from build123d import *

# Parameters (mm, degrees)
F1_DEPTH = 5
F2_DEPTH = 15
F3_D     = 1.25


with BuildPart() as f1:
    # F0 (on Front) → F1 (new body)
    with BuildSketch(Plane.XZ):
        with BuildLine():
            ThreePointArc((6.4951905284, -3.75), (7.2444436972, -1.9411428383), (7.5, 0))
            ThreePointArc((7.5, 0), (5.3033008589, 5.3033008589), (0, 7.5))
            Line((0, 7.5), (0, 0))
            Line((0, 0), (6.4951905284, -3.75))
        make_face()
        with BuildLine():
            Line((0, 0), (0, 7.5))
            ThreePointArc((0, 7.5), (-6.4951905284, 3.75), (-6.4951905284, -3.75))
            Line((-6.4951905284, -3.75), (0, 0))
        make_face()
        with BuildLine():
            ThreePointArc((6, -4.5), (6.2588394759, -4.1324240362), (6.4951905284, -3.75))
            Line((6.4951905284, -3.75), (0, 0))
            Line((0, 0), (-6.4951905284, -3.75))
            ThreePointArc((-6.4951905284, -3.75), (-6.2588394759, -4.1324240362), (-6, -4.5))
            Line((-6, -4.5), (6, -4.5))
        make_face()
    extrude(amount=F1_DEPTH)

    # F0 (on Front) → F2 (join)
    with BuildSketch(Plane.XZ):
        with BuildLine():
            ThreePointArc((0, -7.5), (3.3541019662, -6.7082039325), (6, -4.5))
            Line((6, -4.5), (-6, -4.5))
            ThreePointArc((-6, -4.5), (-3.3541019662, -6.7082039325), (0, -7.5))
        make_face()
        with BuildLine():
            Line((6, -7.5), (6, -4.5))
            ThreePointArc((6, -4.5), (3.3541019662, -6.7082039325), (0, -7.5))
            Line((0, -7.5), (6, -7.5))
        make_face()
        with BuildLine():
            ThreePointArc((0, -7.5), (-3.3541019662, -6.7082039325), (-6, -4.5))
            Line((-6, -4.5), (-6, -7.5))
            Line((-6, -7.5), (0, -7.5))
        make_face()
    extrude(amount=F2_DEPTH)

    # F3 (through all)
    with Locations(Plane(origin=(0, 0, 0), x_dir=(1, 0, 0), z_dir=(0, 1, 0))):
        with Locations((3.4641016151, 2), (-3.4641016151, 2), (0, -4.5)):
            Hole(F3_D / 2)


solid = f1.part
Input: part model. Units: mm. Frame: model coordinates. A direction names the side the tool comes from. Give positions to 0.01 mm unless a question says otherwise; leave off trailing zeros. Write each loop counter-clockwise with the first axis right and the second up, starting at its lowest first coordinate (ties: lowest second). Pieces come first, ordered by that corner, then holes. Notation, with made-up numbers: M 72,-27.75 L 111,-27.75 A6 ccw 111,-20.75 Z; hole C -29,-4 d10. An arc over 180 degrees is marked long. Write item = value, one per line. Start each with the question number.
1) Material intervals for line 1 along X through (y, z) = (-1.25, -1.5); line 2 along X through (y, z) = (-5.5, -6.25); line 3 along Y through (x, z) = (-2.25, 6.5), sorted ascending. Write a range as [from, to].
2) Draft query along Z for faces 1 (the flat face through (0, -10, -4.5)), 2 (the cylindrical face through (-0.596, -2.535, 4.312)), 3 (the flat face through (0, -5, 2)). Return one class per face: +Z half, -Z half, draft (parallel to the pull), parting line (faces both ways), or undercut.
3) Cut plane C-C on z = -2. Return the cut outline in (x, y).
4) Cut plane D-D on y = -7.25. Return the cut outline in (x, z).
5) First-contact query: pin 1 Ø4 at (y, z) = (-3.5, -5) entering from -X; pin 2 Ø2 at (x, z) = (-2.5, 1.5) entering from -Y; pin 3 Ø4 at (y, z) = (-8.5, 4) entering from -X; pin 4 Ø0.9 at (y, z) = (-6.5, -6) entering from +X. Flat tips, straight axial feed; report the tip coordinate or a pass-through.
6) Cut plane A-A on z = 4.5. Return the cut outline in (x, y) (3 decimals).
7) Reachability of faces 4 (the flat face through (6, -7, -6)), 5 (the flat face through (0, 0, 0)), 6 (the flat face through (-6, -7, -6)) from +Z, -Z, +X, -X, +Y, -Y: full face, straight path, thin tool, end or side. Return the list, or none.
8) Cut plane B-B on y = -1.25. Return the cut outline in (x, z) (3 decimals), then the cut area to 3 significant figures.
Solved:
q1.line_1 = [-7.35, -3.84], [-3.09, 3.09], [3.84, 7.35]
q1.line_2 = [-6, 6]
q1.line_3 = [-5, 0]
q2.face_1 = +Z half
q2.face_2 = undercut
q2.face_3 = draft
q3.outline = M -7.23,-5 L -4.09,-5 L -4.09,0 L -7.23,0 Z; M -2.84,-5 L 2.84,-5 L 2.84,0 L -2.84,0 Z; M 4.09,-5 L 7.23,-5 L 7.23,0 L 4.09,0 Z
q4.outline = M -6,-7.5 L 6,-7.5 L 6,-4.5 L -6,-4.5 Z
q5.pin_1 = -6.87
q5.pin_2 = -5
q5.pin_3 = through
q5.pin_4 = 6
q6.outline = M -6,-5 L -0.625,-5 L -0.625,0 L -6,0 Z; M 0.625,-5 L 6,-5 L 6,0 L 0.625,0 Z
q7.face_4 = -Z, +X, +Y, -Y
q7.face_5 = +Z, -Z, +X, -X, +Y
q7.face_6 = -Z, -X, +Y, -Y
q8.outline = M -6,-7.5 L 6,-7.5 L 6,-4.5 A7.5 ccw long -6,-4.5 Z; hole C -3.464,-2 d1.25; hole C 0,4.5 d1.25; hole C 3.464,-2 d1.25
q8.area = 184 mm2
